Could you check a few things on this drawing? It's one solid part, dimensions in mm from its lowest x, y, z. Give positions to 0.01 mm unless a question says otherwise; leave off trailing zeros. Order: outer loops, then holes, each group sorted by start corner. A loop starts at its lowest first (then second) coordinate and runs counter-clockwise, first axis right, second up.
Item 1: If I drill on line 1 along Z through (x, y) = (35.5, 0.5); line 2 along X through (y, z) = (1.9, 16.51); line 3 along X through (y, z) = (1.65, 39.37) (3 decimals), over which ranges is the centre line in solid material (lowest first)?
Item 2: I want a section at D-D, the plane x = 45.5. Write out the boundary of the cut face in (y, z).
Item 3: I want a section at B-B, the plane z = 39.37. Write out the boundary of the cut face in (x, y) (3 decimals).
Item 4: I want a section at A-A, the plane x = 35.56. Write out the boundary of the cut face in (y, z) (3 decimals), then the cut area to 3 significant figures.
Item 5: I want a section at C-C, the plane y = 2.05. Write out the boundary of the cut face in (x, z) (3 decimals).
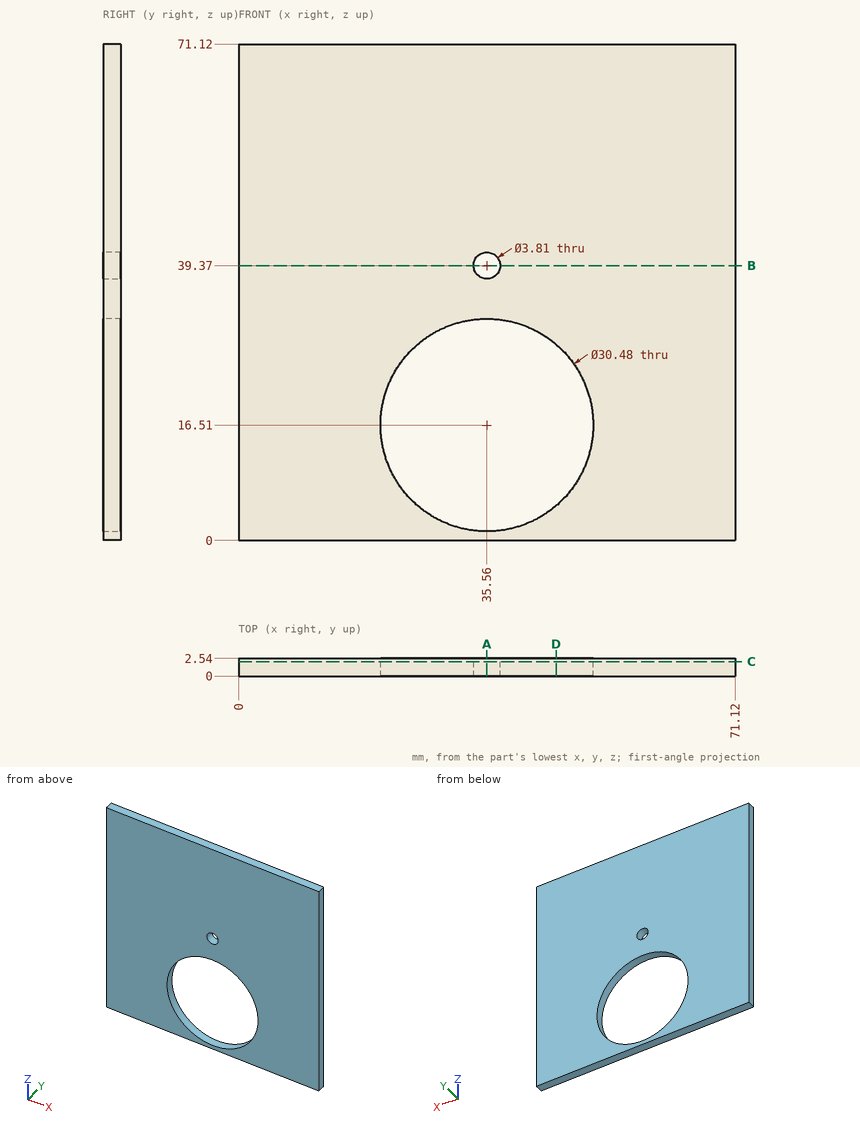
Results list:
1. line 1: z = 0 to 1.27, 31.75 to 37.47, 41.27 to 71.12
1. line 2: x = 0 to 20.32, 50.8 to 71.12
1. line 3: x = 0 to 33.655, 37.465 to 71.12
2. outline: (0, 0) - (2.54, 0) - (2.54, 4.96) - (0, 4.96) - close; (0, 28.06) - (2.54, 28.06) - (2.54, 71.12) - (0, 71.12) - close
3. outline: (0, 0) - (33.655, 0) - (33.655, 2.54) - (0, 2.54) - close; (37.465, 0) - (71.12, 0) - (71.12, 2.54) - (37.465, 2.54) - close
4. outline: (0, 0) - (2.54, 0) - (2.54, 1.27) - (0, 1.27) - close; (0, 31.75) - (2.54, 31.75) - (2.54, 37.465) - (0, 37.465) - close; (0, 41.275) - (2.54, 41.275) - (2.54, 71.12) - (0, 71.12) - close
4. area: 93.5 mm2
5. outline: (0, 0) - (71.12, 0) - (71.12, 71.12) - (0, 71.12) - close; hole circle Ø30.48 at (35.56, 16.51); hole circle Ø3.81 at (35.56, 39.37)
